Source: CAD feature listing. Evaluate the final solid. Frame: model axes, mm. Face numbers are marked on the shaded views. Coordinates: 2 decimals unless noted, no trailing zeros. Order: outer loops, then holes, each group sorted by start corner. A loop starts at its lowest first (then second) coordinate and runs counter-clockwise, first axis right, second up. Notation, with made-up numbers: (42, 40) -> (59, 40) arc R10 ccw to (59, 47) -> close; hole circle Ø6 at (-31.5, -29). An arc over 180 degrees is marked (long way). Write item = value, one per line. Start each with the question number.
Item 1: Ray query, line 1 along Y through (x, z) = (-13.5, 5); line 2 along Z through (x, y) = (-6, 2); line 3 along Y through (x, z) = (19, 15.5). Return the intervals inside material, ascending. Write a range as [from, to].
Item 2: Section query B-B (y = 6). Output: boundary loops of the cut face in (x, z), then the cut area to 3 significant figures.
Item 3: Section query D-D (x = -1.5). Output: boundary loops of the cut face in (y, z), then the cut area to 3 significant figures.
Item 4: Section query A-A (x = 15). Output: boundary loops of the cut face in (y, z), then the cut area to 3 significant figures.
Item 5: Mould query, pull axis Y, two halves, no side actions, for the marked faces 1, 2, 3 and 4. Classes: released by +Y, released by -Y, zero draft, split by the parting line, or undercut.
Item 6: Contact query for flat-ended pins moving along their axis: pin 1 (9 mm diameter, centred on x = 6.5, z = -1, fed in from +Y); pin 2 (4 mm diameter, centred on x = -22.225, z = 24.765, fed in from -Y); pin 3 (1.3 mm diameter, centred on x = 3.5, y = 13.5, fed in from -Z); pin 4 (10 mm diameter, centred on x = 6.5, z = 17, fed in from +Y). Output: stop coordinate, or through.
Item 7: Section query C-C (z = -8). Output: boundary loops of the cut face in (x, y), then the cut area to 3 significant figures.
```python
from build123d import *

# Parameters (mm, degrees)
SKETCH1_W                 = 50.8
SKETCH1_H                 = 55.88
BOSS_EXTRUDE1_DEPTH       = 1.5748
F_4_CLEARANCE_HOLE1_D     = 3.2639
F_4_CLEARANCE_HOLE1_DEPTH = 76.2
F_4_CLEARANCE_HOLE1_TIP   = 0.980574487
SKETCH4_W                 = 38.1
SKETCH4_H                 = 2.54
BOSS_EXTRUDE2_DEPTH       = 11.176
SKETCH5_W                 = 43.18
SKETCH5_H                 = 18.288
BOSS_EXTRUDE3_DEPTH       = 1.5748
SKETCH6_W                 = 9.1694
SKETCH6_H                 = 7.5438
BOSS_EXTRUDE4_DEPTH       = 3.556


with BuildPart() as part:
    # Sketch1 → Boss-Extrude1 (new body)
    with BuildSketch(Plane(origin=(0, 0, 0), x_dir=(1, 0, 0), z_dir=(0, 1, 0))):
        Rectangle(SKETCH1_W, SKETCH1_H)
    extrude(amount=BOSS_EXTRUDE1_DEPTH)

    # #4 Clearance Hole1
    with Locations(Plane(origin=(0, 1.5748, 0), x_dir=(-1, 0, 0), z_dir=(0, 1, 0))):
        with Locations((22.225, 24.765), (22.225, -24.765), (-22.225, -24.765), (-22.225, 24.765)):
            Hole(F_4_CLEARANCE_HOLE1_D / 2, depth=F_4_CLEARANCE_HOLE1_DEPTH)
            with Locations((0, 0, -(F_4_CLEARANCE_HOLE1_DEPTH + F_4_CLEARANCE_HOLE1_TIP / 2))):  # 118° drill point
                Cone(0, F_4_CLEARANCE_HOLE1_D / 2, F_4_CLEARANCE_HOLE1_TIP, mode=Mode.SUBTRACT)

    # Sketch4 → Boss-Extrude2 (add)
    with BuildSketch(Plane(origin=(0, 1.5748, 0), x_dir=(1, 0, 0), z_dir=(0, 1, 0))):
        with Locations((0, -7.62)):
            Rectangle(SKETCH4_W, SKETCH4_H)
        with Locations((0, 7.62)):
            Rectangle(SKETCH4_W, SKETCH4_H)
    extrude(amount=BOSS_EXTRUDE2_DEPTH)

    # Sketch5 → Boss-Extrude3 (add)
    with BuildSketch(Plane(origin=(0, 12.7508, 0), x_dir=(1, 0, 0), z_dir=(0, 1, 0))):
        Rectangle(SKETCH5_W, SKETCH5_H)
    extrude(amount=BOSS_EXTRUDE3_DEPTH)

    # Sketch6 → Boss-Extrude4 (add)
    with BuildSketch(Plane(origin=(0, 14.3256, 0), x_dir=(1, 0, 0), z_dir=(0, 1, 0))):
        with Locations((18.2753, 0)):
            Rectangle(SKETCH6_W, SKETCH6_H)
    extrude(amount=BOSS_EXTRUDE4_DEPTH)


solid = part.part
```
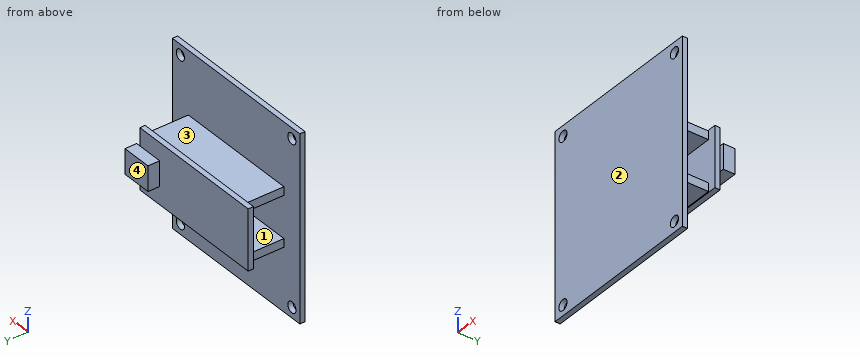
Computed:
q1.line_1 = [0, 1.57], [12.75, 14.33]
q1.line_2 = [-8.89, -6.35], [6.35, 8.89]
q1.line_3 = [0, 1.57]
q2.outline = (-19.05, -8.89) -> (19.05, -8.89) -> (19.05, -6.35) -> (-19.05, -6.35) -> close; (-19.05, 6.35) -> (19.05, 6.35) -> (19.05, 8.89) -> (-19.05, 8.89) -> close
q2.area = 194 mm^2
q3.outline = (0, -27.94) -> (1.57, -27.94) -> (1.57, -8.89) -> (12.75, -8.89) -> (12.75, -9.14) -> (14.33, -9.14) -> (14.33, 9.14) -> (12.75, 9.14) -> (12.75, 8.89) -> (1.57, 8.89) -> (1.57, 27.94) -> (0, 27.94) -> close; hole (1.57, -6.35) -> (12.75, -6.35) -> (12.75, 6.35) -> (1.57, 6.35) -> close
q3.area = 174 mm^2
q4.outline = (0, -27.94) -> (1.57, -27.94) -> (1.57, -8.89) -> (12.75, -8.89) -> (12.75, -9.14) -> (14.33, -9.14) -> (14.33, -3.77) -> (17.88, -3.77) -> (17.88, 3.77) -> (14.33, 3.77) -> (14.33, 9.14) -> (12.75, 9.14) -> (12.75, 8.89) -> (1.57, 8.89) -> (1.57, 27.94) -> (0, 27.94) -> close; hole (1.57, -6.35) -> (12.75, -6.35) -> (12.75, 6.35) -> (1.57, 6.35) -> close
q4.area = 200 mm^2
q5.face_1 = undercut
q5.face_2 = released by -Y
q5.face_3 = undercut
q5.face_4 = released by +Y
q6.pin_1 = 14.33
q6.pin_2 = 0
q6.pin_3 = -9.14
q6.pin_4 = 1.57
q7.outline = (-25.4, 0) -> (25.4, 0) -> (25.4, 1.57) -> (19.05, 1.57) -> (19.05, 12.75) -> (21.59, 12.75) -> (21.59, 14.33) -> (-21.59, 14.33) -> (-21.59, 12.75) -> (-19.05, 12.75) -> (-19.05, 1.57) -> (-25.4, 1.57) -> close
q7.area = 574 mm^2
